Autodesk Inventor part; units mm, degrees
ref_plane "YZ Plane" through (0, 0, 0) normal (1, 0, 0) x (0, 1, 0)
ref_plane "XZ Plane" through (0, 0, 0) normal (0, 1, 0) x (-1, 0, 0)
ref_plane "XY Plane" through (0, 0, 0) normal (0, 0, 1) x (1, 0, 0)
sketch "main" plane through (0, 0, 0) normal (0, 0, 1) x (1, 0, 0)
  circle A0 centre (16.9271, 1.4076) radius 2.1844
  arc A1 (-15.8903, 3.592) -> (-15.8903, -0.7768) centre (-15.8903, 1.4076) ccw
  arc A2 (16.9271, -4.9424) -> (16.9271, 7.7576) centre (16.9271, 1.4076) ccw
  arc A3 (-15.8903, 7.7576) -> (-15.8903, -4.9424) centre (-15.8903, 1.4076) ccw
  line L0 (-15.8903, 7.7576) -> (16.9271, 7.7576)
  line L1 (16.9271, -4.9424) -> (-15.8903, -4.9424)
  arc A4 (0.4077, -0.7768) -> (0.4077, 3.592) centre (0.4077, 1.4076) ccw
  line L2 (-15.8903, 3.592) -> (0.4077, 3.592)
  line L3 (0.4077, -0.7768) -> (-15.8903, -0.7768)
  point P0 (-1.0706, 1.6197)
  dimension "d0" = 12.7
  dimension "d1" = 12.7
  dimension "d3" = 32.8174
  dimension "d4" = 4.3688
  dimension "d5" = 4.3688
sketch "Sketch1" plane through (0, 0, 0) normal (0, 0, 1) x (1, 0, 0)
  circle A0 centre (32.8174, 0) radius 2.1844
  arc A1 (0, 2.1844) -> (0, -2.1844) centre (0, 0) ccw
  arc A2 (32.8174, -6.35) -> (32.8174, 6.35) centre (32.8174, 0) ccw
  arc A3 (0, 6.35) -> (0, -6.35) centre (0, 0) ccw
  line L0 (0, 6.35) -> (32.8174, 6.35)
  line L1 (32.8174, -6.35) -> (0, -6.35)
  arc A4 (16.298, -2.1844) -> (16.298, 2.1844) centre (16.298, 0) ccw
  line L2 (0, 2.1844) -> (16.298, 2.1844)
  line L3 (16.298, -2.1844) -> (0, -2.1844)
extrude "Extrusion1" add sketch "Sketch1" along normal blind 1.5875
properties part number "Hardstop Gusset" material "Acetal Resin, White"
The listing builds one solid part. Answer for the finished solid, in the listing's coordinates (mm). A direction names the side the tool comes from. Give positions to 0.01 mm unless a question says otherwise; leave off trailing zeros. Order: outer loops, then holes, each group sorted by start corner. A loop starts at its lowest first (then second) coordinate and runs counter-clockwise, first axis right, second up.
1) Find section B-B on y = 0. Write down the section's boundary in (x, z), then the cut area to 3 significant figures.
Reported:
outline: (-6.35, 0) - (-2.18, 0) - (-2.18, 1.59) - (-6.35, 1.59) - close; (18.48, 0) - (30.63, 0) - (30.63, 1.59) - (18.48, 1.59) - close; (35, 0) - (39.17, 0) - (39.17, 1.59) - (35, 1.59) - close
area: 32.5 mm2
2) Consider line 1 along Y through (x, z) = (14, 0.1); line 2 along X through (y, z) = (-1.75, 1.25); line 3 along X through (y, z) = (-1.25, 0.6). Determine where each line is inside the solid, lowest interval first.
Reported:
line 1: y = -6.35 to -2.18, 2.18 to 6.35
line 2: x = -6.1 to -1.31, 17.61 to 31.51, 34.12 to 38.92
line 3: x = -6.23 to -1.79, 18.09 to 31.03, 34.61 to 39.04
3) For faces 1 (the face through (8, -2.184, 1)), 2 (the face through (16, 6.35, 1)), determine the directions among +Z, -Z, +X, -X, +Y, -Y from which every point of the face is accessible in a straight line to the end or side of a thin tool.
Reported:
face 1: +Z, -Z
face 2: +Z, -Z, +X, -X, +Y
4) Determine the mould class of faces 3 (the face through (16, -3, 0)), 4 (the face through (-6.35, -0.14, 0.78)), 5 (the face through (8, 2.184, 1)), 6 (the face through (34.835, 0.837, 0.783)) for opening direction Y: pulls with the +Y half, pulls with the -Y half, needs draft (parallel to the pull), parting line crosses it, or undercut.
Reported:
face 3: needs draft
face 4: parting line crosses it
face 5: undercut
face 6: undercut
5) Find section C-C on y = -5. Write down the section's boundary in (x, z), then the cut area to 3 significant figures.
Reported:
outline: (-3.91, 0) - (36.73, 0) - (36.73, 1.59) - (-3.91, 1.59) - close
area: 64.5 mm2
6) Find section D-D on y = -3. Write down the section's boundary in (x, z), then the cut area to 3 significant figures.
Reported:
outline: (-5.6, 0) - (38.41, 0) - (38.41, 1.59) - (-5.6, 1.59) - close
area: 69.9 mm2
7) Find section A-A on z = 1.25. Write down the section's boundary in (x, y).
Reported:
outline: (0, -6.35) - (32.82, -6.35) arc R6.35 ccw to (32.82, 6.35) - (0, 6.35) arc R6.35 ccw to start; hole (0, -2.18) - (16.3, -2.18) arc R2.18 ccw to (16.3, 2.18) - (0, 2.18) arc R2.18 ccw to start; hole circle Ø4.37 at (32.82, 0)
